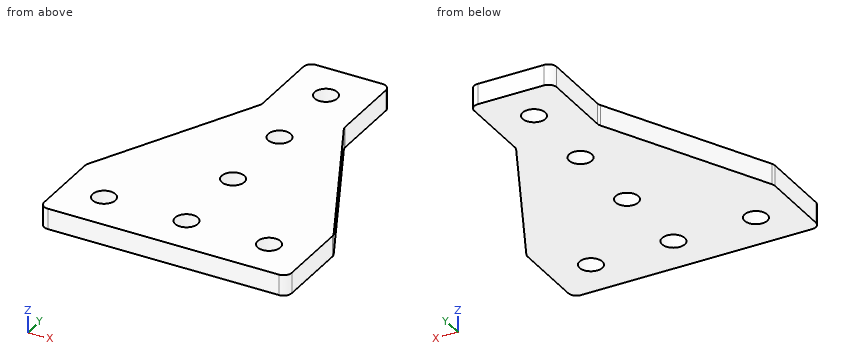
Autodesk Inventor part; units mm, degrees
ref_plane "YZ Plane" through (0, 0, 0) normal (1, 0, 0) x (0, 1, 0)
ref_plane "XZ Plane" through (0, 0, 0) normal (0, 1, 0) x (-1, 0, 0)
ref_plane "XY Plane" through (0, 0, 0) normal (0, 0, 1) x (1, 0, 0)
sketch "Sketch2" plane through (0, 0, 0) normal (0, 0, 1) x (1, 0, 0)
  line L0 (0, 0) -> (0, 20) construction
  line L1 (0, 20) -> (0, 40) construction
  line L2 (0, 40) -> (0, 60) construction
  line L3 (0, 0) -> (20, 0) construction
  line L4 (0, 0) -> (-20, 0) construction
  line L5 (-30, 10) -> (-10, 50)
  line L6 (-10, 50) -> (-10, 70)
  line L7 (-10, 70) -> (10, 70)
  line L8 (10, 70) -> (10, 50)
  line L9 (10, 50) -> (30, 10)
  line L10 (30, 10) -> (30, -10)
  line L11 (30, -10) -> (-30, -10)
  line L12 (-30, -10) -> (-30, 10)
  line L13 (0, 0) -> (0, -10) construction
  line L14 (0, 70) -> (0, 60) construction
  dimension "d0" = 20
  dimension "d1" = 10
  dimension "d2" = 20
  dimension "d3" = 60
  dimension "d4" = 10
  dimension "d5" = 20
extrude "Extrusion1" add sketch "Sketch2" along normal blind 5
hole "Hole1" at (0, 40, 0) at (0, 20, 0) at (0, 60, 0) at (-20, 0, 0) at (0, 0, 0) at (20, 0, 0) direction (0, 0, 1) diameter 5.5 end through all
fillet "Fillet1" radius 2 8 edges at (-10, 70, 2.5) (-30, 10, 2.5) (-30, -10, 2.5) (30, -10, 2.5) (30, 10, 2.5) (10, 70, 2.5) (10, 50, 2.5) (-10, 50, 2.5)
properties part number "8060T"
Here's how the part is built. I have some questions about the finished solid (model axes, mm). Round coordinates to 2 decimals unless told otherwise and drop trailing zeros. Order: outer loops, then holes, each group sorted by start corner. A loop starts at its lowest first (then second) coordinate and runs counter-clockwise, first axis right, second up. Notation, with made-up numbers: M -6,21 L 11,21 A10 cw 11,36 Z; hole C 24.5,18.25 d9. An arc over 180 degrees is marked long. Return JSON: item names as keys, results as strings. Group by question number.
1. If we section it at C-C on z = 4.1: List the corners of the cut face in (x, y) for me, then the cut area to 3 significant figures.
2. If we section it at B-B on x = 20: List the corners of the cut face in (y, z) for me.
3. I'm going to push flat-ended pins straight in: pin 1 Ø1.5 at (y, z) = (40, 3) entering from +X (3 decimals); pin 2 Ø2.5 at (y, z) = (57.5, 2) entering from +X; pin 3 Ø1.5 at (y, z) = (62.5, 2.5) entering from -X. Where does each tip first touch, or does it pass through?
4. If we section it at D-D on y = 0: List the corners of the cut face in (x, z) for me, then the cut area to 4 significant figures.
5. If we section it at A-A on y = 40: List the corners of the cut face in (x, z) for me, then the cut area to 4 significant figures.
6. Please list where these lines run through material, in increasing order: probe 1 along Y at (x, z) = (0, 1.4); probe 2 along X at (y, z) = (60, 2.6); probe 3 along Y at (x, z) = (-1, 3.7).
Reply:
{
 "1": {"outline": "M -30,-8 A2 ccw -28,-10 L 28,-10 A2 ccw 30,-8 L 30,9.53 A2 ccw 29.79,10.42 L 10.21,49.58 A2 cw 10,50.47 L 10,68 A2 ccw 8,70 L -8,70 A2 ccw -10,68 L -10,50.47 A2 cw -10.21,49.58 L -29.79,10.42 A2 ccw -30,9.53 Z; hole C -20,0 d5.5; hole C 0,0 d5.5; hole C 0,20 d5.5; hole C 0,40 d5.5; hole C 0,60 d5.5; hole C 20,0 d5.5", "area": "3,050 mm^2"},
 "2": {"outline": "M -10,0 L -2.75,0 L -2.75,5 L -10,5 Z; M 2.75,0 L 30,0 L 30,5 L 2.75,5 Z"},
 "3": {"pin 1": "x = 15.375", "pin 2": "x = 10", "pin 3": "x = -10"},
 "4": {"outline": "M -30,0 L -22.75,0 L -22.75,5 L -30,5 Z; M -17.25,0 L -2.75,0 L -2.75,5 L -17.25,5 Z; M 2.75,0 L 17.25,0 L 17.25,5 L 2.75,5 Z; M 22.75,0 L 30,0 L 30,5 L 22.75,5 Z", "area": "217.5 mm^2"},
 "5": {"outline": "M -15,0 L -2.75,0 L -2.75,5 L -15,5 Z; M 2.75,0 L 15,0 L 15,5 L 2.75,5 Z", "area": "122.5 mm^2"},
 "6": {"probe 1": "-10 to -2.75, 2.75 to 17.25, 22.75 to 37.25, 42.75 to 57.25, 62.75 to 70", "probe 2": "-10 to -2.75, 2.75 to 10", "probe 3": "-10 to -2.56, 2.56 to 17.44, 22.56 to 37.44, 42.56 to 57.44, 62.56 to 70"}
}
